from build123d import *

# Parameters (mm, degrees)
SKETCH1_R           = 5.08
SKETCH1_R_2         = 3.175
BOSS_EXTRUDE1_DEPTH = 7
FILLET6_R           = 38.1
FILLET9_R           = 7.62
FILLET10_R          = 7.62
FILLET11_R          = 3.81
FILLET12_R          = 20.32
FILLET13_R          = 38.1
SKETCH2_R           = 6.067865864
CUT_EXTRUDE1_DEPTH  = 2.54


with BuildPart() as part:
    # Sketch1 → Boss-Extrude1 (new body)
    with BuildSketch(Plane(origin=(0, 0, 0), x_dir=(1, 0, 0), z_dir=(0, 1, 0))):
        with BuildLine():
            Line((-88.899351346, 69.85), (88.899351346, 69.85))
            ThreePointArc((88.899351346, 69.85), (114.3, 0), (88.899351346, -69.85))
            Line((88.899351346, -69.85), (-88.899351346, -69.85))
            ThreePointArc((-88.899351346, -69.85), (-114.3, 0), (-88.899351346, 69.85))
        make_face()
        with Locations(Location((0, -25.4, 0), (0, 0, 270))):
            Circle(SKETCH1_R, mode=Mode.SUBTRACT)
        with Locations(Location((-21.997045256, 12.7, 0), (0, 0, 270))):
            Circle(SKETCH1_R, mode=Mode.SUBTRACT)
        with Locations(Location((21.997045256, 12.7, 0), (0, 0, 270))):
            Circle(SKETCH1_R, mode=Mode.SUBTRACT)
        with Locations(Location((-88.560044244, 48.26, 0), (0, 0, 270))):
            Circle(SKETCH1_R_2, mode=Mode.SUBTRACT)
        with Locations(Location((-88.560044244, -48.26, 0), (0, 0, 90))):
            Circle(SKETCH1_R_2, mode=Mode.SUBTRACT)
        with Locations(Location((88.560044244, -48.26, 0), (0, 0, 270))):
            Circle(SKETCH1_R_2, mode=Mode.SUBTRACT)
        with Locations(Location((88.560044244, 48.26, 0), (0, 0, 90))):
            Circle(SKETCH1_R_2, mode=Mode.SUBTRACT)
        Polygon((-60.864265129, 62.23), (60.864265129, 62.23), (33.730665032, 26.578259891), (-33.730665032, 26.578259891), align=None, mode=Mode.SUBTRACT)
        with BuildLine():
            Line((-66.2189372, -57.15), (-10.16, -57.15))
            Line((-10.16, -57.15), (-10.16, -25.362104437))
            Line((-10.16, -25.362104437), (-69.836388427, 53.048688207))
            ThreePointArc((-69.836388427, 53.048688207), (-83.989429266, 28.185034179), (-88.9, 0))
            ThreePointArc((-88.9, 0), (-83.022483728, -30.743101298), (-66.2189372, -57.15))
        make_face(mode=Mode.SUBTRACT)
        with BuildLine():
            Line((10.16, -25.362104437), (10.16, -57.15))
            Line((10.16, -57.15), (66.2189372, -57.15))
            ThreePointArc((66.2189372, -57.15), (83.022483728, -30.743101298), (88.9, 0))
            ThreePointArc((88.9, 0), (83.989429266, 28.185034179), (69.836388427, 53.048688207))
            Line((69.836388427, 53.048688207), (10.16, -25.362104437))
        make_face(mode=Mode.SUBTRACT)
    extrude(amount=BOSS_EXTRUDE1_DEPTH)

    # Fillet6
    fillet6_edges = [part.edges().sort_by_distance(p)[0] for p in [
        (-66.2189372, 3.5, 57.15),
        (66.2189372, 3.5, 57.15),
        (-88.899351346, 3.5, -69.85),
        (88.899351346, 3.5, -69.85),
        (88.899351346, 3.5, 69.85),
        (-88.899351346, 3.5, 69.85),
    ]]
    fillet(fillet6_edges, radius=FILLET6_R)

    # Fillet9
    fillet9_edges = [part.edges().sort_by_distance(p)[0] for p in [
        (-10.16, 3.5, 57.15),
        (10.16, 3.5, 57.15),
    ]]
    fillet(fillet9_edges, radius=FILLET9_R)

    # Fillet10
    fillet10_edges = [part.edges().sort_by_distance(p)[0] for p in [
        (-69.836388427, 3.5, -53.048688207),
        (69.836388427, 3.5, -53.048688207),
    ]]
    fillet(fillet10_edges, radius=FILLET10_R)

    # Fillet11
    fillet11_edges = [part.edges().sort_by_distance(p)[0] for p in [
        (60.864265129, 3.5, -62.23),
        (-60.864265129, 3.5, -62.23),
    ]]
    fillet(fillet11_edges, radius=FILLET11_R)

    # Fillet12
    fillet12_edges = [part.edges().sort_by_distance(p)[0] for p in [
        (33.730665032, 3.5, -26.578259891),
        (-33.730665032, 3.5, -26.578259891),
    ]]
    fillet(fillet12_edges, radius=FILLET12_R)

    # Fillet13
    fillet13_edges = [part.edges().sort_by_distance(p)[0] for p in [
        (-10.16, 3.5, 25.362104437),
        (10.16, 3.5, 25.362104437),
    ]]
    fillet(fillet13_edges, radius=FILLET13_R)

    # Sketch2 → Cut-Extrude1 (cut)
    with BuildSketch(Plane(origin=(0, 7, 0), x_dir=(1, 0, 0), z_dir=(0, 1, 0))):
        with Locations(Location((0, 0, 0), (0, 0, 270))):
            Circle(SKETCH2_R)
    extrude(amount=-CUT_EXTRUDE1_DEPTH, mode=Mode.SUBTRACT)


solid = part.part
Could you check a few things on this model? Use its own coordinates, in mm. A direction names the side the tool comes from. Coordinates: 2 decimals unless noted, no trailing zeros. Order: outer loops, then holes, each group sorted by start corner. A loop starts at its lowest first (then second) coordinate and runs counter-clockwise, first axis right, second up. Notation, with made-up numbers: (-34.75, -37.75) - (-28.75, -37.75) arc R30 ccw to (-28.75, -5.75) - close; hole circle Ø11 at (-12, 33.25). An arc over 180 degrees is marked (long way). Answer in a Markdown table with one row per item. Add a question column.
(1) If we section it at A-A, the plane x = 0: Please give me the cut outline in (y, z), then the cut area to 3 significant figures.
(2) If we section it at B-B, the plane z = -59.5: Please give me the cut outline in (x, y).
(3) If we mould it in two halves opening along Z, with no side actions, what happens to faces 1 (the face through (-26.956, 3.451, -13.801)), 2 (the face through (-88.9, 3.55, 64.03)), 3 (the face through (2, 0, -1)), 4 (the face through (-114.298, 3.451, 0.71))? For each: released by +Z, released by -Z, zero draft, split by the parting line, or undercut.
(4) If we section it at C-C, the plane z = 25.4: Please give me the cut outline in (x, y), then the cut area to 3 significant figures.
(5) If we section it at D-D, the plane x = -35: Please give me the cut outline in (y, z).
(6) Will these pins go through, and if not, where does the flat tip stop? pin 1 (3 mm diameter, centred on y = 4.5, z = 48.5, fed in from -X); pin 2 (3.5 mm diameter, centred on x = -2.5, z = 1.5, fed in from +Y); pin 3 (1 mm diameter, centred on x = 84.5, y = 3.5, fed in from +Z).
(7) I need wall thicknesses on L1, parallel to X at y = 5.5, z = -48.26; L2, parallel to Z at x = 9, y = 0.75; L3, parallel to X at y = 1.5, z = 39. Which ranges of each line are inside material? Lowest first, please.
(8) On a 3-axis mill with a long thin cutter (end or side, diameter ignored), from which of +Z, -Z, +X, -X, +Y, -Y can I reach the whole of each face in a straight line? I mean faces 5 (the face through (12.214, 3.549, 25.872)), 6 (the face through (-3.692, 5.748, -4.815)), 7 (the face through (114.298, 3.451, -0.71)). Say none if no direction works.
Results are:
| question | item | result |
|---|---|---|
| 1 | outline | (0, -69.85) - (7, -69.85) - (7, -62.23) - (0, -62.23) - close; (0, -26.58) - (7, -26.58) - (7, -6.07) - (4.46, -6.07) - (4.46, 6.07) - (7, 6.07) - (7, 20.32) - (0, 20.32) - close; (0, 30.48) - (7, 30.48) - (7, 69.85) - (0, 69.85) - close |
| 1 | area | 626 mm2 |
| 2 | outline | (-94.77, 0) - (-56.83, 0) - (-56.83, 7) - (-94.77, 7) - close; (56.83, 0) - (94.77, 0) - (94.77, 7) - (56.83, 7) - close |
| 3 | face 1 | undercut |
| 3 | face 2 | released by +Z |
| 3 | face 3 | zero draft |
| 3 | face 4 | split by the parting line |
| 4 | outline | (-111.29, 0) - (-84.94, 0) - (-84.94, 7) - (-111.29, 7) - close; (-12.38, 0) - (-5.08, 0) - (-5.08, 7) - (-12.38, 7) - close; (5.08, 0) - (12.38, 0) - (12.38, 7) - (5.08, 7) - close; (84.94, 0) - (111.29, 0) - (111.29, 7) - (84.94, 7) - close |
| 4 | area | 471 mm2 |
| 5 | outline | (0, -69.85) - (7, -69.85) - (7, -62.23) - (0, -62.23) - close; (0, -30.04) - (7, -30.04) - (7, -7.28) - (0, -7.28) - close; (0, 57.15) - (7, 57.15) - (7, 69.85) - (0, 69.85) - close |
| 6 | pin 1 | stops at x = -103.62 |
| 6 | pin 2 | stops at y = 4.46 |
| 6 | pin 3 | stops at z = 66.63 |
| 7 | L1 | x = -103 to -91.74, -85.39 to -50.23, 50.23 to 85.39, 91.74 to 103 |
| 7 | L2 | z = -69.85 to -62.23, -26.58 to 69.85 |
| 7 | L3 | x = -107.07 to -79.05, -10.16 to 10.16, 79.05 to 107.07 |
| 8 | face 5 | +Y, -Y |
| 8 | face 6 | +Y |
| 8 | face 7 | +X, +Y, -Y |
